Input: part model. Units: mm. Frame: model coordinates. Face numbers are marked on the shaded views. A direction names the side the tool comes from. Give positions to 0.01 mm unless a question says otherwise; leave off trailing zeros. Write each loop counter-clockwise with the first axis right and the second up, starting at its lowest first coordinate (ties: lowest second). Pieces come first, ordered by that corner, then holes.
```python
from build123d import *

# Parameters (mm, degrees)
SKETCH2_OUTSIDE_W  = 43.314
SKETCH2_OUTSIDE_H  = 43.314
CUT_EXTRUDE1_DEPTH = 10
SKETCH3_R          = 1.3
CUT_EXTRUDE2_DEPTH = 3
SKETCH5_R          = 9
SKETCH5_R_2        = 7
CUT_EXTRUDE3_DEPTH = 4.3


with BuildPart() as part:
    # Sketch1 → Revolve1 (revolve)
    with BuildSketch(Plane.XY):
        with BuildLine():
            Line((-2.5, 10), (-2.5, 0))
            Line((-2.5, 0), (-9, 0))
            Line((-9, 0), (-9, 16))
            Line((-9, 16), (1, 16))
            ThreePointArc((1, 16), (1.707106781, 15.707106781), (2, 15))
            Line((2, 15), (2, 11))
            ThreePointArc((2, 11), (1.707106781, 10.292893219), (1, 10))
            Line((1, 10), (-2.5, 10))
        make_face()
    revolve(axis=Axis((0, 0, 0), (-1, 0, 0)))

    # Sketch2 outside → Cut-Extrude1 (cut, through all)
    with BuildSketch(Plane(origin=(0, 0, 0), x_dir=(0, 0, -1), z_dir=(1, 0, 0))):
        Rectangle(SKETCH2_OUTSIDE_W, SKETCH2_OUTSIDE_H)
        with BuildLine():
            Line((5, 13.25), (-5, 13.25))
            ThreePointArc((-5, 13.25), (-5.707106781, 12.957106781), (-6, 12.25))
            Line((-6, 12.25), (-6, 10.656570743))
            ThreePointArc((-6, 10.656570743), (-6.119937614, 10.181712663), (-6.450980392, 9.820761273))
            ThreePointArc((-6.450980392, 9.820761273), (0, -11.75), (6.450980392, 9.820761273))
            ThreePointArc((6.450980392, 9.820761273), (6.119937614, 10.181712663), (6, 10.656570743))
            Line((6, 10.656570743), (6, 12.25))
            ThreePointArc((6, 12.25), (5.707106781, 12.957106781), (5, 13.25))
        make_face(mode=Mode.SUBTRACT)
    extrude(amount=-CUT_EXTRUDE1_DEPTH, mode=Mode.SUBTRACT)

    # Sketch3 → Cut-Extrude2 (cut, through all)
    with BuildSketch(Plane(origin=(0, 0, 0), x_dir=(0, 0, -1), z_dir=(1, 0, 0))):
        with Locations((-11, 7.829080757)):
            Circle(SKETCH3_R)
        with Locations((11, 7.829080757)):
            Circle(SKETCH3_R)
        with Locations((0, -13.501648251)):
            Circle(SKETCH3_R)
        with BuildLine():
            Line((-12.664898978, 5.629114116), (-13.210413813, 6.664678663))
            ThreePointArc((-13.210413813, 6.664678663), (-13.492769962, 7.995992047), (-13.035445505, 9.277777778))
            ThreePointArc((-13.035445505, 9.277777778), (0, -16), (13.035445505, 9.277777778))
            ThreePointArc((13.035445505, 9.277777778), (13.492769962, 7.995992047), (13.210413813, 6.664678663))
            Line((13.210413813, 6.664678663), (12.664898978, 5.629114116))
            ThreePointArc((12.664898978, 5.629114116), (12.551470751, 5.223399463), (12.615189348, 4.806973861))
            ThreePointArc((12.615189348, 4.806973861), (11.930739874, -6.317234051), (3.114633748, -13.135792957))
            ThreePointArc((3.114633748, -13.135792957), (2.619659949, -13.420790107), (2.361421665, -13.930236303))
            ThreePointArc((2.361421665, -13.930236303), (0, -15.901648251), (-2.361421665, -13.930236303))
            ThreePointArc((-2.361421665, -13.930236303), (-2.619659949, -13.420790107), (-3.114633748, -13.135792957))
            ThreePointArc((-3.114633748, -13.135792957), (-11.930739874, -6.317234051), (-12.615189348, 4.806973861))
            ThreePointArc((-12.615189348, 4.806973861), (-12.551470751, 5.223399463), (-12.664898978, 5.629114116))
        make_face()
    extrude(amount=CUT_EXTRUDE2_DEPTH, mode=Mode.SUBTRACT)

    # Sketch4 → Cut-Revolve1 (revolve, cut)
    with BuildSketch(Plane.XY, mode=Mode.PRIVATE) as cut_revolve1_sk:
        with BuildLine():
            Line((-2.5, -1), (-8, -1))
            Line((-8, -1), (-8, -9))
            ThreePointArc((-8, -9), (-7.707106781, -9.707106781), (-7, -10))
            Line((-7, -10), (-2.5, -10))
            Line((-2.5, -10), (-2.5, -1))
        make_face()
    revolve(cut_revolve1_sk.sketch.rotate(Axis((2, -1, 0), (-1, 0, 0)), 180), axis=Axis((2, -1, 0), (-1, 0, 0)), mode=Mode.SUBTRACT)  # turned: the seam where the file's is

    # Sketch5 → Cut-Extrude3 (cut)
    with BuildSketch(Plane(origin=(0, 13.25, 0), x_dir=(-1, 0, 0), z_dir=(0, 1, 0))):
        with Locations((12, 0)):
            Circle(SKETCH5_R)
        with Locations((12, 0)):
            Circle(SKETCH5_R_2, mode=Mode.SUBTRACT)
    extrude(amount=-CUT_EXTRUDE3_DEPTH, mode=Mode.SUBTRACT)


solid = part.part
```
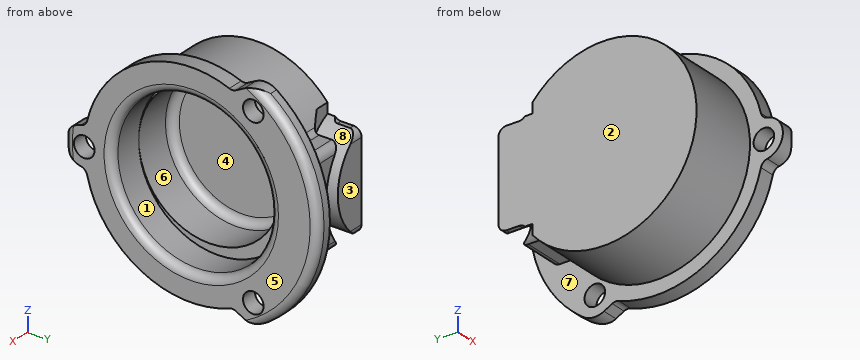
Q1. Mould query, pull axis Y, two halves, no side actions, for the marked faces 1, 2, 3 and 4. Classes: +Y half, -Y half, draft (parallel to the pull), parting line (faces both ways), or undercut.
Q2. Pin query (flat end, axial travel): pin 1 (1.6 mm diameter, centred on y = 7.83, z = -11, fed in from +X); pin 2 (0.5 mm diameter, centred on x = -9, y = 11.5, fed in from +Z); pin 3 (2.5 mm diameter, centred on x = -3, z = 1, fed in from +Y); pin 4 (1.3 mm diameter, centred on x = -2.5, y = 11, fed in from -Z). Return the tip coordinate at first contact, or that it passes through.
Q3. Material intervals for line 1 along Z through (x, y) = (-1.5, 0); line 2 along X through (y, z) = (-5, -1.75); line 3 along X through (y, z) = (8, -9.5), sorted ascending.
Q4. Section A-A, the plane x = 0.5. Return the cut outline in (y, z).
Q5. Access query for the marked faces 5, 6, 7 and 8. Directions: +Z, -Z, +X, -X, +Y, -Y. A direction counts if a zero-diameter tool reaches every point of the face in a straight line with its end or side. Return the directions, or none.
Solutions:
1. face 1: undercut
1. face 2: draft
1. face 3: +Y half
1. face 4: undercut
2. pin 1: passes through
2. pin 2: stops at z = 6
2. pin 3: stops at y = 13.25
2. pin 4: stops at z = -6.05
3. line 1: z = -11.75 to -10, 10 to 11.75
3. line 2: x = -9 to -8
3. line 3: x = 0 to 2
4. outline: (-13.93, -2.36) arc R1 cw to (-13.14, -3.11) arc R13.5 ccw to (4.81, -12.62) arc R1 cw to (5.63, -12.66) - (6.66, -13.21) arc R2.5 ccw to (9.28, -13.04) arc R16 ccw to (9.28, 13.04) arc R2.5 ccw to (6.66, 13.21) - (5.63, 12.66) arc R1 cw to (4.81, 12.62) arc R13.5 ccw to (-13.14, 3.11) arc R1 cw to (-13.93, 2.36) arc R2.4 ccw to start; hole circle Ø2.6 at (-13.5, 0); hole circle Ø20 at (0, 0); hole circle Ø2.6 at (7.83, -11); hole circle Ø2.6 at (7.83, 11)
5. face 5: +Z, -Z, +X, +Y, -Y
5. face 6: +X
5. face 7: -X
5. face 8: +Y
